Work out the finished part from the listing and answer in its coordinate system (mm). Face numbers are marked on the shaded views. Coordinates: 2 decimals unless noted, no trailing zeros. Loops run counter-clockwise (first coordinate to the right, second up) from the corner with the lowest first, then second, coordinate; pieces in that order, holes last. Notation, with made-up numbers: (-34, 7.5) -> (-17, 7.5) arc R27 ccw to (-17, 46.5) -> close; hole circle Ø11 at (66.25, 69). An arc over 180 degrees is marked (long way). One line per question, with ' | ' between items.
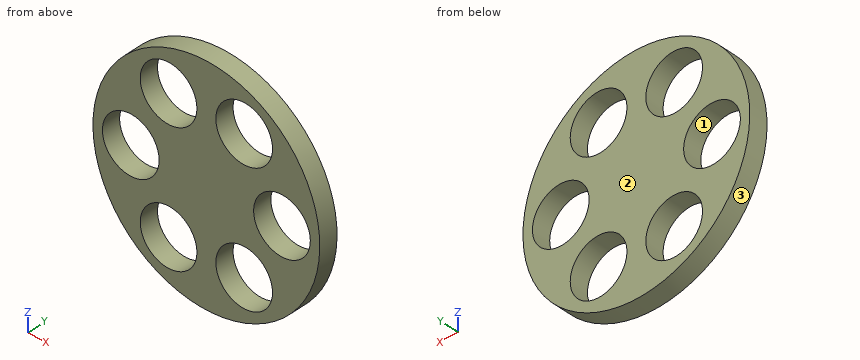
```python
from build123d import *

# Parameters (mm, degrees)
ESQUISSE1_R                      = 60
BOSS_EXTRU_1_DEPTH               = 5
ESQUISSE2_R                      = 15
ENL_V_MAT_EXTRU_1_DEPTH          = 86
R_P_TITION_START                 = -5
R_P_TITION_CIRCULAIRE1_OUTLINE_R = 15
R_P_TITION_CIRCULAIRE1_DEPTH     = 10


# Read off the part's stored shape, not the designer's step: Répétition circulaire1
with BuildPart() as part:
    # Esquisse1 → Boss.-Extru.1 (new, symmetric)
    with BuildSketch(Plane(origin=(0, 0, 0), x_dir=(1, 0, 0), z_dir=(0, 1, 0))):
        with Locations(Location((0, 0, 0), (0, 0, 270))):
            Circle(ESQUISSE1_R)
    extrude(amount=BOSS_EXTRU_1_DEPTH, both=True)

    # Esquisse2 → Enlèv. mat.-Extru.1 (cut, symmetric)
    with BuildSketch(Plane(origin=(0, 0, 0), x_dir=(1, 0, 0), z_dir=(0, 1, 0))):
        with Locations(Location((40, 0, 0), (0, 0, 270))):
            Circle(ESQUISSE2_R)
    extrude(amount=ENL_V_MAT_EXTRU_1_DEPTH, both=True, mode=Mode.SUBTRACT)

    # Répétition circulaire1 outline → Répétition circulaire1 (cut)
    with BuildSketch(Plane(origin=(0, 0, 0), x_dir=(1, 0, 0), z_dir=(0, 1, 0)).offset(R_P_TITION_START)):
        with Locations((20, 34.641016151)):
            Circle(R_P_TITION_CIRCULAIRE1_OUTLINE_R)
        with Locations((-20, 34.641016151)):
            Circle(R_P_TITION_CIRCULAIRE1_OUTLINE_R)
        with Locations((-40, 0)):
            Circle(R_P_TITION_CIRCULAIRE1_OUTLINE_R)
        with Locations((-20, -34.641016151)):
            Circle(R_P_TITION_CIRCULAIRE1_OUTLINE_R)
        with Locations((20, -34.641016151)):
            Circle(R_P_TITION_CIRCULAIRE1_OUTLINE_R)
    extrude(amount=R_P_TITION_CIRCULAIRE1_DEPTH, mode=Mode.SUBTRACT)


solid = part.part
```
1) Find section C-C (y = 3.25). Write down the section's boundary in (x, z).
Check values:
outline: circle Ø120 at (0, 0); hole circle Ø30 at (-40, 0); hole circle Ø30 at (-20, -34.64); hole circle Ø30 at (-20, 34.64); hole circle Ø30 at (20, -34.64); hole circle Ø30 at (20, 34.64); hole circle Ø30 at (40, 0)
2) Find the intervals of material crossed by line 1 along X through (y, z) = (1.25, 0); line 2 along X through (y, z) = (1.5, -12.5); line 3 along Z through (x, y) = (17.5, 2.5), in increasing order.
Check values:
line 1: x = -60 to -55, -25 to 25, 55 to 60 | line 2: x = -58.68 to -48.29, -31.71 to 31.71, 48.29 to 58.68 | line 3: z = -57.39 to -49.43, -19.85 to 19.85, 49.43 to 57.39
3) Find section A-A (x = -49.5). Write down the section's boundary in (y, z), plus the area to 3 significant figures.
Check values:
outline: (-5, -33.91) -> (5, -33.91) -> (5, -11.61) -> (-5, -11.61) -> close; (-5, 11.61) -> (5, 11.61) -> (5, 33.91) -> (-5, 33.91) -> close | area: 446 mm^2
4) Find section D-D (x = 19). Write down the section's boundary in (y, z).
Check values:
outline: (-5, -56.91) -> (5, -56.91) -> (5, -49.61) -> (-5, -49.61) -> close; (-5, -19.67) -> (5, -19.67) -> (5, 19.67) -> (-5, 19.67) -> close; (-5, 49.61) -> (5, 49.61) -> (5, 56.91) -> (-5, 56.91) -> close
5) Flat-ended cylindrical pins translate along their axes: pin 1 (5 mm diameter, centred on x = 39, y = -0.5, fed in from -Z); pin 2 (1.5 mm diameter, centred on x = 30, y = -1, fed in from -Z); pin 3 (1.5 mm diameter, centred on x = -35.5, y = -1, fed in from -Z). Find the tip coordinate at first contact, or state that the pin passes through.
Check values:
pin 1: stops at z = -47.62 | pin 2: stops at z = -52.39 | pin 3: stops at z = -48.91
6) Find section B-B (z = 6.5). Write down the section's boundary in (x, y).
Check values:
outline: (-59.65, -5) -> (-53.52, -5) -> (-53.52, 5) -> (-59.65, 5) -> close; (-26.48, -5) -> (26.48, -5) -> (26.48, 5) -> (-26.48, 5) -> close; (53.52, -5) -> (59.65, -5) -> (59.65, 5) -> (53.52, 5) -> close
7) The mould has two halves that part along Z. Classify the marked faces 1, 2 and 3: released by +Z, released by -Z, zero draft, split by the parting line, or undercut.
Check values:
face 1: undercut | face 2: zero draft | face 3: split by the parting line
